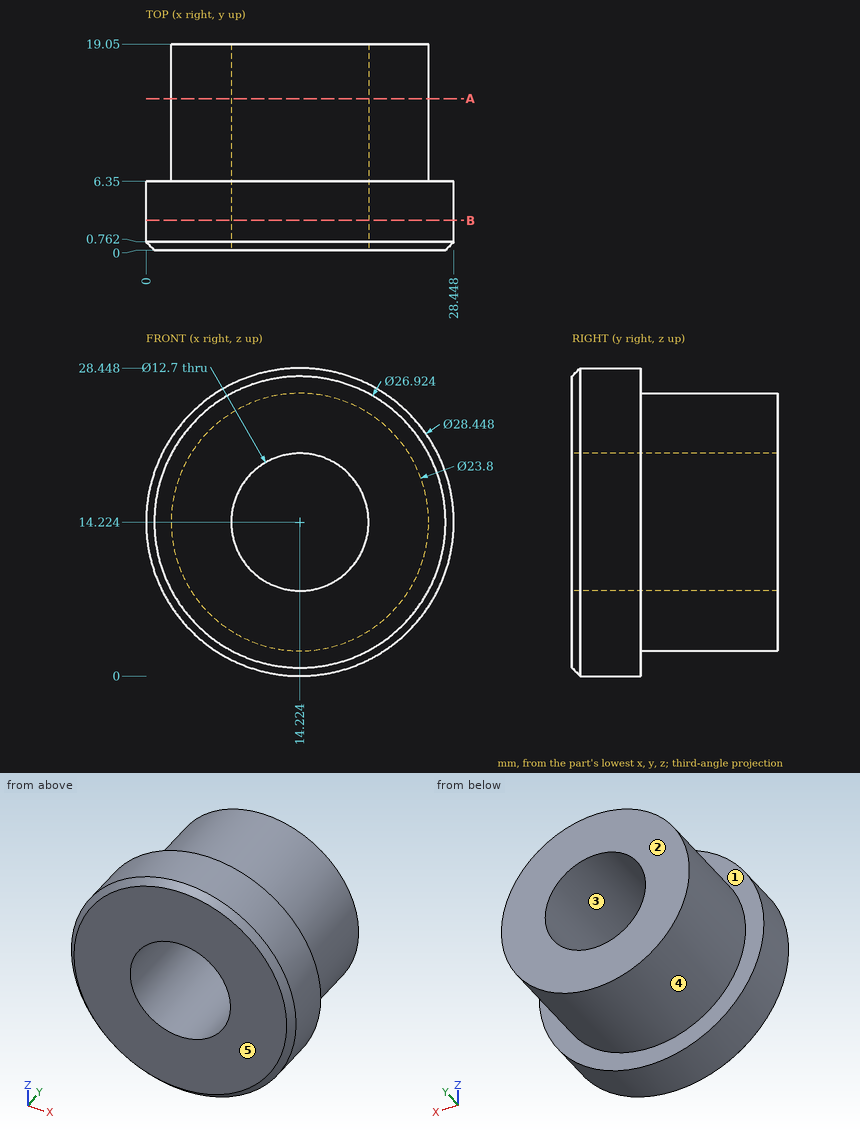
The figure shows three views and two pictorial views of one solid part (mm, origin at its lowest corner). Answer the questions. A direction names the side the tool comes from. Round coordinates to 2 decimals unless told otherwise and drop trailing zeros. Order: outer loops, then holes, each group sorted by start corner. A loop starts at its lowest first (then second) coordinate and runs counter-clockwise, first axis right, second up. Notation, with made-up numbers: M 52,89 L 78,89 A18 ccw 78,106 Z; hole C 47,-6 d10. An arc over 180 degrees is marked long. Answer in a Markdown table with one row per item. Add a question column.
1) Which of the six approach directions +Z, -Z, +X, -X, +Y, -Y give full straight-line access (tool end or side, diameter ignored) to the marked faces 1 and 2?
2) The part is cut by section B-B on y = 2.75. Determine the outline of the cut face in (x, z).
3) Flat-ended cylindrical pins translate along their axes: pin 1 Ø2 at (y, z) = (16.5, 23.5) entering from -X; pin 2 Ø7.5 at (x, z) = (14.224, 14.224) entering from -Y; pin 3 Ø5 at (y, z) = (7, 10) entering from +X; pin 4 Ø2 at (x, y) = (4, 3.5) entering from +Z. Find the tip coordinate at first contact, or state that the pin passes through.
4) The part is cut by section A-A on y = 14. Determine the outline of the cut face in (x, z), plus the area to 3 significant figures.
5) Consider line 1 along Z through (x, y) = (18, 5.75); line 2 along X through (y, z) = (15.25, 11) (1 decimal); line 3 along X through (y, z) = (17.75, 11.75). Determine where each line is inside the solid, lowest interval first. Write a range as from..to.
6) Determine the mould class of the marked faces 3, 4 and 5 for opening direction Z: pulls with the +Z half, pulls with the -Z half, needs draft (parallel to the pull), parting line crosses it, or undercut.
Findings below:
| question | item | result |
|---|---|---|
| 1 | face 1 | +Y |
| 1 | face 2 | +Z, -Z, +X, -X, +Y |
| 2 | outline | C 14.22,14.22 d28.45; hole C 14.22,14.22 d12.7 |
| 3 | pin 1 | stops at x = 5.67 |
| 3 | pin 2 | passes through |
| 3 | pin 3 | stops at x = 28.33 |
| 3 | pin 4 | stops at z = 25.05 |
| 4 | outline | C 14.22,14.22 d23.8; hole C 14.22,14.22 d12.7 |
| 4 | area | 318 mm² |
| 5 | line 1 | z = 0.51..9.12, 19.33..27.94 |
| 5 | line 2 | x = 2.8..8.8, 19.7..25.7 |
| 5 | line 3 | x = 2.58..8.38, 20.07..25.86 |
| 6 | face 3 | undercut |
| 6 | face 4 | parting line crosses it |
| 6 | face 5 | needs draft |
